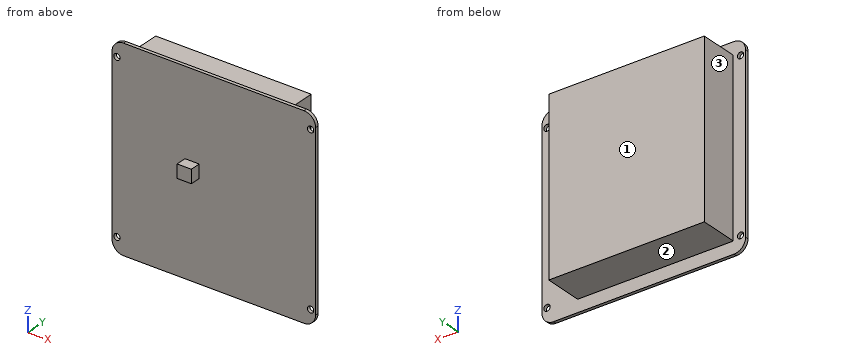
```python
from build123d import *

# Parameters (mm, degrees)
SKETCH1_W           = 99.910000078
SKETCH1_H           = 96.25
SKETCH1_R           = 1.55
BOSS_EXTRUDE1_DEPTH = 1.6
FILLET1_R           = 5.7
SKETCH2_W           = 76.33
SKETCH2_H           = 84.11
BOSS_EXTRUDE2_DEPTH = 18.9
SKETCH3_W           = 6.96
SKETCH3_H           = 6.55
BOSS_EXTRUDE3_DEPTH = 5.15


with BuildPart() as part:
    # Sketch1 → Boss-Extrude1 (new body)
    with BuildSketch(Plane(origin=(0, 0, 0), x_dir=(1, 0, 0), z_dir=(0, 1, 0))):
        Rectangle(SKETCH1_W, SKETCH1_H)
        with Locations((-47.5, 40.75)):
            Circle(SKETCH1_R, mode=Mode.SUBTRACT)
        with Locations((47.5, 40.75)):
            Circle(SKETCH1_R, mode=Mode.SUBTRACT)
        with Locations((-47.5, -40.75)):
            Circle(SKETCH1_R, mode=Mode.SUBTRACT)
        with Locations((47.5, -40.75)):
            Circle(SKETCH1_R, mode=Mode.SUBTRACT)
    extrude(amount=BOSS_EXTRUDE1_DEPTH)

    # Fillet1
    fillet1_edges = [part.edges().sort_by_distance(p)[0] for p in [
        (-49.955000039, 0.8, -48.125),
        (49.955000039, 0.8, -48.125),
        (49.955000039, 0.8, 48.125),
        (-49.955000039, 0.8, 48.125),
    ]]
    fillet(fillet1_edges, radius=FILLET1_R)

    # Sketch2 → Boss-Extrude2 (add)
    with BuildSketch(Plane(origin=(0, 1.6, 0), x_dir=(1, 0, 0), z_dir=(0, 1, 0))):
        with Locations((-5.730000039, 0)):
            Rectangle(SKETCH2_W, SKETCH2_H)
    extrude(amount=BOSS_EXTRUDE2_DEPTH)

    # Sketch3 → Boss-Extrude3 (add)
    with BuildSketch(Plane.XZ):
        with Locations((-10.615000039, 2.95)):
            Rectangle(SKETCH3_W, SKETCH3_H)
    extrude(amount=BOSS_EXTRUDE3_DEPTH)


solid = part.part
```
The model under review builds one solid part; all positions refer to its coordinate system, in mm. Face numbers are marked on the shaded views. A direction names the side the tool comes from. Coordinates: 2 decimals unless noted, no trailing zeros. Write each loop counter-clockwise with the first axis right and the second up, starting at its lowest first coordinate (ties: lowest second). Pieces come first, ordered by that corner, then holes.
1) We need section D-D on x = 47.5. State the section outline as (y, z) points, then the cut area to 3 significant figures.
2) We need section C-C on x = -16. State the section outline as (y, z) points (3 decimals), then the cut area to 3 significant figures.
3) We need section A-A on z = 40.75. State the section outline as (x, y) points (3 decimals), then the cut area to 3 significant figures.
4) Clearance check with flat-ended pins moving along their axes: pin 1 Ø2.5 at (y, z) = (-1.5, 4.5) entering from -X (3 decimals); pin 2 Ø5.5 at (x, y) = (-17.5, 13.5) entering from +Z (3 decimals); pin 3 Ø4 at (y, z) = (-4, 2) entering from +X (3 decimals); pin 4 Ø1.9 at (x, z) = (-47.5, 40.75) entering from +Y. State where each tip first meets the part, or that it passes through.
5) Machinability: for the marked faces 1, 2 and 3, which of the approach directions +Z, -Z, +X, -X, +Y, -Y give a long, thin tool a straight path to every point of the face, cutting with its end or side? Answer none if there is none.
6) We need section B-B on z = 5. State the section outline as (x, y) points (3 decimals), then the cut area to 3 significant figures.
7) To check wall thickness, follow probe 1 along X at (y, z) = (0.45, 40.75) (3 decimals); probe 2 along Z at (x, y) = (47.5, 1.2); probe 3 along X at (y, z) = (10.5, -28) (3 decimals). State the ranges of each line that lie inside material, in increasing order.
Answer list:
1. outline: (0, -47.11) - (1.6, -47.11) - (1.6, -42.3) - (0, -42.3) - close; (0, -39.2) - (1.6, -39.2) - (1.6, 39.2) - (0, 39.2) - close; (0, 42.3) - (1.6, 42.3) - (1.6, 47.11) - (0, 47.11) - close
1. area: 141 mm2
2. outline: (0, -48.125) - (1.6, -48.125) - (1.6, -42.055) - (20.5, -42.055) - (20.5, 42.055) - (1.6, 42.055) - (1.6, 48.125) - (0, 48.125) - close
2. area: 1,740 mm2
3. outline: (-49.955, 0) - (-49.05, 0) - (-49.05, 1.6) - (-49.955, 1.6) - close; (-45.95, 0) - (45.95, 0) - (45.95, 1.6) - (32.435, 1.6) - (32.435, 20.5) - (-43.895, 20.5) - (-43.895, 1.6) - (-45.95, 1.6) - close; (49.05, 0) - (49.955, 0) - (49.955, 1.6) - (49.05, 1.6) - close
3. area: 1,590 mm2
4. pin 1: stops at x = -14.095
4. pin 2: stops at z = 42.055
4. pin 3: stops at x = -7.135
4. pin 4: passes through
5. face 1: +Z, -Z, +X, -X, +Y
5. face 2: -Z, +X, -X, +Y
5. face 3: +Z, -Z, -X, +Y
6. outline: (-49.955, 0) - (-14.095, 0) - (-14.095, -5.15) - (-7.135, -5.15) - (-7.135, 0) - (49.955, 0) - (49.955, 1.6) - (32.435, 1.6) - (32.435, 20.5) - (-43.895, 20.5) - (-43.895, 1.6) - (-49.955, 1.6) - close
6. area: 1,640 mm2
7. probe 1: x = -49.955 to -49.05, -45.95 to 45.95, 49.05 to 49.955
7. probe 2: z = -47.11 to -42.3, -39.2 to 39.2, 42.3 to 47.11
7. probe 3: x = -43.895 to 32.435
